Geometry check sheet. Reference: the model listing, model coordinates, mm. Face numbers are marked on the shaded views. A direction names the side the tool comes from. Round coordinates to 2 decimals unless told otherwise and drop trailing zeros. Loops run counter-clockwise (first coordinate to the right, second up) from the corner with the lowest first, then second, coordinate; pieces in that order, holes last. Notation, with made-up numbers: (50, -9.75) - (61, -9.75) arc R21 cw to (61, 14.25) - close; hole circle Ø5 at (-25.75, 52). An arc over 180 degrees is marked (long way). Answer as CSV lines item,"result". Start each with the question number.
1) Depth check by flat-ended pin: P1, Ø4, axis at y = 5.5, z = -12.5, coming from the +X side; P2, Ø2, axis at x = 0, z = 14, coming from the -Y side; P3, Ø2, axis at y = 5, z = 7.5, coming from the +X side; P4, Ø4, axis at y = 5, z = 8, coming from the -X side. Enter the tip coordinate at first touch or a pass-through.
2) Access from +Z, -Z, +X, -X, +Y, -Y to the whole of each face (thin tool, end or side, straight path). Record for the marked faces 1, 2 and 3.
3) Cross-section at C-C on y = 8. Record the boundary of the cut face in (x, z), and give its area (3 significant figures).
4) Cross-section at D-D on z = 0. Record the boundary of the cut face in (x, y).
5) Cross-section at A-A on x = -1. Record the boundary of the cut face in (y, z), and give its area (3 significant figures).
6) Thickness scan on line 1 along Z through (x, y) = (0, 2.75); line 2 along X through (y, z) = (4.25, 7.5); line 3 along X through (y, z) = (6, 0). Record the ranges inside material, lowest first.
7) Draft check along Z on the marked faces 4, 5 and 6. Enter one of: released by +Z, released by -Z, zero draft, split by the parting line, or undercut.
8) Cross-section at B-B on z = 7. Record the boundary of the cut face in (x, y).
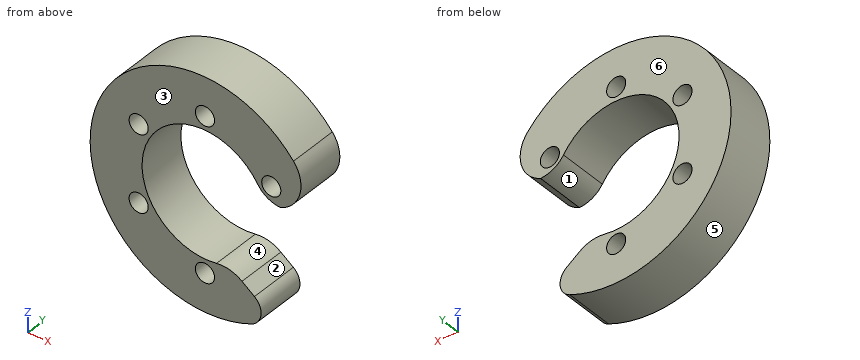
from build123d import *

# Parameters (mm, degrees)
SKETCH_1_R               = 21
EXTRUDE_1_DEPTH          = 9
HOLE_WIZARD_1_D          = 3.5
PATTERN_CIRCULAR_1_COUNT = 6
HOLE_WIZARD_2_D          = 23
SKETCH_7_W               = 20
SKETCH_7_H               = 8
CUT_EXTRUDE_1_DEPTH      = 10
FILLET_1_R               = 5
FILLET_2_R               = 6
CUT_EXTRUDE_2_DEPTH      = 10
FILLET_3_R               = 6
FILLET_4_R               = 3


with BuildPart() as part:
    # 草图1 → 凸台-拉伸1 (new body)
    with BuildSketch(Plane(origin=(0, 0, 0), x_dir=(1, 0, 0), z_dir=(0, 1, 0))):
        with Locations(Location((0, 0, 0), (0, 0, 270))):
            Circle(SKETCH_1_R)
    extrude(amount=EXTRUDE_1_DEPTH)

    # 孔1 (through all)
    with Locations(Plane(origin=(0, 9, 0), x_dir=(1, 0, 0), z_dir=(0, 1, 0))):
        with Locations((0, 14)):
            hole_wizard_1 = Hole(HOLE_WIZARD_1_D / 2)

    # 阵列(圆周)1: 孔1 ×6 about axis
    pattern_circular_1_axis = Axis((0, 0, 0), (0, 1, 0))
    for i in range(1, PATTERN_CIRCULAR_1_COUNT):
        add(hole_wizard_1.rotate(pattern_circular_1_axis, i * 360 / PATTERN_CIRCULAR_1_COUNT), mode=Mode.SUBTRACT)

    # 孔2 (through all)
    with Locations(Plane(origin=(0, 9, 0), x_dir=(1, 0, 0), z_dir=(0, 1, 0))):
        with Locations((0, 0)):
            Hole(HOLE_WIZARD_2_D / 2)

    # 草图7 → 切除-拉伸1 (cut)
    with BuildSketch(Plane.XZ):
        with Locations((14, 0)):
            Rectangle(SKETCH_7_W, SKETCH_7_H)
    extrude(amount=-CUT_EXTRUDE_1_DEPTH, mode=Mode.SUBTRACT)

    # 圆角1
    fillet_1_edges = [part.edges().sort_by_distance(p)[0] for p in [
        (10.781929326, 4.5, -4),
        (10.781929326, 4.5, 4),
    ]]
    fillet(fillet_1_edges, radius=FILLET_1_R)

    # 圆角2
    # the kernel refuses this fillet: 6 mm, written as the material it takes off along each edge
    with BuildSketch(Plane(origin=(20.615528128, 34.925810939, 4), x_dir=(-1, 0, 0), z_dir=(0, -1, 0))) as fillet_2_piece_1:
        with BuildLine():
            CenterArc((9.052881986, -5.555376193), FILLET_2_R, 112.196140843, 107.374202327)
            Line((4.427823529, -9.37752667), (4.33532236, -9.45396968))
            ThreePointArc((4.33532236, -9.45396968), (1.517440537, -5.017618885), (-0.117803018, -0.022857143))
            Line((-0.117803018, -0.022857143), (0, 0.12))
            ThreePointArc((0, 0.12), (3.393105721, 0.12), (6.740878031, 0.111107524))
            Line((6.740878031, 0.111107524), (6.786211442, 0))
        make_face()
    extrude(amount=60.851621878, mode=Mode.SUBTRACT)
    with BuildSketch(Plane(origin=(20.615528128, 34.925810939, -4), x_dir=(-0.42697059114477015, 0, -0.9042655109521127), z_dir=(0, -1, 0))) as fillet_2_piece_2:
        with BuildLine():
            CenterArc((8.888849465, -5.814226697), FILLET_2_R, 75.705116129, 107.374202327)
            Line((2.897512711, -6.136536957), (2.777685976, -6.142983162))
            ThreePointArc((2.777685976, -6.142983162), (1.340244494, -3.11950495), (-0.108511861, -0.051236471))
            Line((-0.108511861, -0.051236471), (-0.029629498, 0.116284534))
            ThreePointArc((-0.029629498, 0.116284534), (5.185162188, 0.770206559), (10.399953874, 0.116284534))
            Line((10.399953874, 0.116284534), (10.370324376, 0))
        make_face()
    extrude(amount=60.851621878, mode=Mode.SUBTRACT)

    # 草图8 → 切除-拉伸2 (cut)
    with BuildSketch(Plane(origin=(0, 0, 0), x_dir=(-1, 0, 0), z_dir=(0, -1, 0))):
        Polygon((1.25741602, 6.455059929), (-16.607431005, 19.620253888), (-25.506127326, 7.544940071), (-7.641280301, -5.620253888), align=None)
    extrude(amount=-CUT_EXTRUDE_2_DEPTH, mode=Mode.SUBTRACT)

    # 圆角3
    fillet_3_edges = [part.edges().sort_by_distance(p)[0] for p in [
        (4.400672865, 4.5, -10.624691917),
    ]]
    fillet(fillet_3_edges, radius=FILLET_3_R)

    # 圆角4
    fillet_4_edges = [part.edges().sort_by_distance(p)[0] for p in [
        (12.68916526, 4.5, -16.732754854),
    ]]
    fillet(fillet_4_edges, radius=FILLET_4_R)


solid = part.part
Answer block:
1,P1,"stops at x = 9.54"
1,P2,"passes through"
1,P3,"stops at x = 17.47"
1,P4,"stops at x = -20.12"
2,face 1,"+Y, -Y"
2,face 2,"+X, +Y, -Y"
2,face 3,"+Z, -Z, +X, -X, -Y"
3,outline,"(2.11, -11.3) arc R11.5 cw (long way) to (9.64, 6.27) arc R5 ccw to (13.83, 4) arc R6 ccw to (16.19, 13.38) arc R21 ccw (long way) to (8.48, -19.21) arc R3 ccw to (9.05, -14.05) - (6.77, -12.37) arc R6 ccw to start; hole circle Ø3.5 at (-12.12, -7); hole circle Ø3.5 at (-12.12, 7); hole circle Ø3.5 at (0, -14); hole circle Ø3.5 at (0, 14); hole circle Ø3.5 at (12.12, 7)"
3,area,"700 mm^2"
4,outline,"(-21, 0) - (-11.5, 0) - (-11.5, 9) - (-21, 9) - close"
5,outline,"(0, -20.98) - (9, -20.98) - (9, -15.44) - (0, -15.44) - close; (0, -12.56) - (9, -12.56) - (9, -11.46) - (0, -11.46) - close; (0, 11.46) - (9, 11.46) - (9, 12.56) - (0, 12.56) - close; (0, 15.44) - (9, 15.44) - (9, 20.98) - (0, 20.98) - close"
5,area,"120 mm^2"
6,line 1,"z = -21 to -15.75, -12.25 to -11.5, 11.5 to 12.25, 15.75 to 21"
6,line 2,"x = -19.62 to -13.8, -10.45 to -8.72, 8.72 to 10.45, 13.8 to 17.2"
6,line 3,"x = -21 to -11.5"
7,face 4,"undercut"
7,face 5,"split by the parting line"
7,face 6,"zero draft"
8,outline,"(-19.8, 0) - (-13.87, 0) - (-13.87, 9) - (-19.8, 9) - close; (-10.37, 0) - (-9.12, 0) - (-9.12, 9) - (-10.37, 9) - close; (9.12, 0) - (10.37, 0) - (10.37, 9) - (9.12, 9) - close; (13.87, 0) - (16.99, 0) - (16.99, 9) - (13.87, 9) - close"
